Autodesk Fusion 360 part; units mm, degrees
sketch "Sketch1" plane through (0, 0, 0) normal (0, 0, 1) x (1, 0, 0)
  line L0 (0, 0) -> (-48, 0)
  line L1 (-48, 0) -> (-48, 48)
  line L2 (-48, 48) -> (0, 48)
  line L3 (0, 48) -> (0, 0)
  dimension "d1" = 48
  dimension "d2" = 48
extrude "Extrude1" add sketch "Sketch1" along normal blind 10
sketch "Sketch2" plane through (0, 0, 10) normal (0, 0, 1) x (-1, 0, 0)
  line L0 (0, -48) -> (48, -48)
  line L1 (48, -48) -> (48, 0)
  line L2 (48, 0) -> (0, 0)
  line L3 (0, 0) -> (0, -48)
  line L4 (34.25, -13.75) -> (13.75, -13.75)
  line L5 (13.75, -13.75) -> (13.75, -34.25)
  line L6 (13.75, -34.25) -> (34.25, -34.25)
  line L7 (34.25, -34.25) -> (34.25, -13.75)
  line L8 (34.25, -13.75) -> (13.75, -34.25) construction
  line L9 (13.75, -13.75) -> (34.25, -34.25) construction
  point P0 (24, -24)
  dimension "d5" = 20.5
  dimension "d6" = 20.5
extrude "Extrude2" cut sketch "Sketch2" against normal blind 7 contours L4 L5 L6 L7
sketch "Sketch3" plane through (0, 0, 10) normal (0, 0, 1) x (-1, 0, 0)
  line L0 (13.75, -13.75) -> (34.25, -13.75)
  line L1 (34.25, -13.75) -> (34.25, -34.25)
  line L2 (34.25, -34.25) -> (13.75, -34.25)
  line L3 (13.75, -34.25) -> (13.75, -13.75)
  line L4 (0, -48) -> (48, -48)
  line L5 (48, -48) -> (48, 0)
  line L6 (48, 0) -> (0, 0)
  line L7 (0, 0) -> (0, -48)
sketch "Sketch4" plane through (0, 0, 0) normal (1, 0, 0) x (0, 1, 0)
  line L0 (0, 0) -> (48, 0)
  line L1 (48, 0) -> (48, 10)
  line L2 (48, 10) -> (0, 10)
  line L3 (0, 10) -> (0, 0)
  line L4 (0, 10) -> (18, 10)
  line L5 (18, 10) -> (18, 6.5)
  line L6 (18, 6.5) -> (0, 6.5)
  line L7 (0, 6.5) -> (0, 10)
  circle A0 centre (18, 6.5) radius 2
  dimension "d9" = 18
  dimension "d10" = 3.5
  dimension "d11" = 4
extrude "Extrude3" cut sketch "Sketch4" against normal blind 15 contours L5 L6 A0 | L5 L6 A0
fillet "Fillet1" radius 4 1 edges at (0, 48, 5)
fillet "Fillet2" radius 4 1 edges at (0, 0, 5)
fillet "Fillet3" radius 4 2 edges at (-48, 48, 5) (-48, 0, 5)
sketch "Sketch5" plane through (0, 0, 10) normal (0, 0, 1) x (-1, 0, 0)
  line L0 (13.75, -13.75) -> (11.25, -13.75)
  line L1 (11.25, -13.75) -> (11.25, -11.25)
  line L2 (11.25, -11.25) -> (13.75, -11.25)
  line L3 (13.75, -11.25) -> (13.75, -13.75)
  line L4 (11.25, -11.25) -> (36.75, -11.25)
  line L5 (36.75, -11.25) -> (36.75, -36.75)
  line L6 (36.75, -36.75) -> (11.25, -36.75)
  line L7 (11.25, -36.75) -> (11.25, -11.25)
  circle A0 centre (36.75, -36.75) radius 1.6
  circle A1 centre (11.25, -36.75) radius 1.6
  circle A2 centre (11.25, -11.25) radius 1.6
  circle A3 centre (36.75, -11.25) radius 1.6
  point P0 (13.75, -13.75)
  dimension "d20" = 2.5
  dimension "d21" = 2.5
  dimension "d22" = 25.5
  dimension "d23" = 25.5
  dimension "d24" = 3.2
  dimension "d25" = 3.2
  dimension "d26" = 3.2
  dimension "d27" = 3.2
extrude "Extrude4" cut sketch "Sketch5" against normal blind 2 contours L1 L2 L4 L7 A2 | L1 L2 L4 L7 A2 | L6 L7 A1 | L6 L7 A1 | L4 L5 A3 | L4 L5 A3 | L5 L6 A0 | L5 L6 A0
sketch "Sketch6" plane through (0, 0, 0) normal (0, 0, -1) x (1, 0, 0)
  arc A0 (-44, 0) -> (-48, -4) centre (-44, -4) ccw
  line L0 (-48, -4) -> (-48, -44)
  arc A1 (-48, -44) -> (-44, -48) centre (-44, -44) ccw
  line L1 (-44, -48) -> (-4, -48)
  arc A2 (-4, -48) -> (0, -44) centre (-4, -44) ccw
  line L2 (0, -44) -> (0, -4)
  arc A3 (0, -4) -> (-4, 0) centre (-4, -4) ccw
  line L3 (-4, 0) -> (-44, 0)
  line L4 (0, 0) -> (-4, 0)
  line L5 (0, -4) -> (0, 0)
  circle A4 centre (-4, -44) radius 1.5
  circle A5 centre (-44, -44) radius 1.5
  circle A6 centre (-44, -4) radius 1.5
  circle A7 centre (-4, -4) radius 1.5
  dimension "d30" = 4
  dimension "d31" = 40
  dimension "d33" = 3
  dimension "d34" = 3
  dimension "d35" = 3
  dimension "d36" = 3
extrude "Extrude5" add sketch "Sketch6" along normal blind 2 contours A4 | A5 | A6 | A7
sketch "Sketch7" plane through (0, 0, 10) normal (0, 0, 1) x (-1, 0, 0)
  line L0 (0, 0) -> (4, 0)
  line L1 (4, 0) -> (4, -4)
  line L2 (4, -4) -> (0, -4)
  line L3 (0, -4) -> (0, 0)
  line L4 (4, -4) -> (44, -4)
  line L5 (44, -4) -> (44, -44)
  line L6 (44, -44) -> (4, -44)
  line L7 (4, -44) -> (4, -4)
  circle A0 centre (4, -4) radius 1.6
  circle A1 centre (44, -4) radius 1.6
  circle A2 centre (4, -44) radius 1.6
  circle A3 centre (44, -44) radius 1.6
  dimension "d39" = 4
  dimension "d40" = 4
  dimension "d41" = 40
  dimension "d42" = 40
  dimension "d43" = 3.2
  dimension "d44" = 3.2
  dimension "d45" = 3.2
  dimension "d46" = 3.2
extrude "Extrude6" cut sketch "Sketch7" against normal blind 2 contours L1 L4 A0 | L1 L2 A0 | L2 L7 A0 | L4 L7 A0 | L4 L5 A1 | L4 L5 A1 | L6 L7 A2 | L6 L7 A2 | L5 L6 A3 | L5 L6 A3
extrude "Extrude7" cut 4 faces at (-44.3721, 3.7344, -2) (-4.5584, 4.2485, -2) (-4.4413, 44.3401, -2) (-43.9601, 44.4654, -2) along direction (0, 0, 1) blind 2
sketch "Sketch8" plane through (0, 0, 0) normal (0, 0, -1) x (1, 0, 0)
  arc A0 (-44, 0) -> (-48, -4) centre (-44, -4) ccw
  line L0 (-48, -4) -> (-48, -44)
  arc A1 (-48, -44) -> (-44, -48) centre (-44, -44) ccw
  line L1 (-44, -48) -> (-4, -48)
  arc A2 (-4, -48) -> (0, -44) centre (-4, -44) ccw
  line L2 (0, -44) -> (0, -4)
  arc A3 (0, -4) -> (-4, 0) centre (-4, -4) ccw
  line L3 (-4, 0) -> (-44, 0)
  line L4 (0, 0) -> (-4, 0)
  line L5 (-4, 0) -> (-4, -4)
  line L6 (-4, -4) -> (0, -4)
  line L7 (0, -4) -> (0, 0)
  line L8 (-4, -4) -> (-44, -4)
  line L9 (-44, -4) -> (-44, -44)
  line L10 (-44, -44) -> (-4, -44)
  line L11 (-4, -44) -> (-4, -4)
  circle A4 centre (-24, -4) radius 1.5
  circle A5 centre (-24, -44) radius 1.5
  circle A6 centre (-4, -24) radius 1.5
  circle A7 centre (-44, -24) radius 1.5
  dimension "d51" = 4
  dimension "d52" = 40
  dimension "d53" = 40
  dimension "d54" = 3
  dimension "d55" = 3
  dimension "d56" = 3
  dimension "d57" = 3
extrude "Extrude8" add sketch "Sketch8" along normal blind 2 contours L8 A4 | L8 A4 | L11 A6 | L11 A6 | L9 A7 | L9 A7 | L10 A5 | L10 A5
sketch "Sketch9" plane through (0, 0, 10) normal (0, 0, 1) x (-1, 0, 0)
  circle A0 centre (4, -4) radius 1.7
  dimension "d60" = 3.4
extrude "Extrude9" cut sketch "Sketch9" against normal blind 2
sketch "Sketch10" plane through (0, 0, 10) normal (0, 0, 1) x (-1, 0, 0)
  circle A0 centre (4, -44) radius 1.7
  arc A1 (0, -44) -> (4, -48) centre (4, -44) ccw
  dimension "d63" = 3.4
extrude "Extrude10" cut sketch "Sketch10" against normal blind 2
sketch "Sketch11" plane through (0, 0, 10) normal (0, 0, 1) x (-1, 0, 0)
  circle A0 centre (44, -4) radius 1.7
  dimension "d66" = 3.4
extrude "Extrude11" cut sketch "Sketch11" against normal blind 2
sketch "Sketch12" plane through (0, 0, 10) normal (0, 0, 1) x (-1, 0, 0)
  circle A0 centre (44, -44) radius 1.7
  dimension "d69" = 3.4
extrude "Extrude12" cut sketch "Sketch12" against normal blind 2
sketch "Sketch13" plane through (0, 0, 10) normal (0, 0, 1) x (-1, 0, 0)
  circle A0 centre (11.25, -11.25) radius 1.7
  circle A1 centre (11.25, -11.25) radius 1.6
  dimension "d72" = 3.4
extrude "Extrude13" cut sketch "Sketch13" against normal blind 2
sketch "Sketch14" plane through (0, 0, 10) normal (0, 0, 1) x (-1, 0, 0)
  circle A0 centre (36.75, -11.25) radius 1.7
  circle A1 centre (36.75, -11.25) radius 1.6
  dimension "d75" = 3.4
extrude "Extrude14" cut sketch "Sketch14" against normal blind 2
sketch "Sketch15" plane through (0, 0, 10) normal (0, 0, 1) x (-1, 0, 0)
  circle A0 centre (36.75, -36.75) radius 1.7
  circle A1 centre (36.75, -36.75) radius 1.6
  dimension "d78" = 3.4
extrude "Extrude15" cut sketch "Sketch15" against normal blind 2
sketch "Sketch16" plane through (0, 0, 10) normal (0, 0, 1) x (-1, 0, 0)
  circle A0 centre (11.25, -36.75) radius 1.7
  circle A1 centre (11.25, -36.75) radius 1.6
  dimension "d81" = 3.4
extrude "Extrude16" cut sketch "Sketch16" against normal blind 2
Part model, mm, in its own coordinate system. A direction names the side the tool comes from. Round coordinates to 2 decimals unless told otherwise and drop trailing zeros. Loops run counter-clockwise (first coordinate to the right, second up) from the corner with the lowest first, then second, coordinate; pieces in that order, holes last. Notation, with made-up numbers: (69.5, 67) -> (74.5, 67) arc R10 cw to (74.5, 71) -> close; hole circle Ø3 at (-38.75, 42). An arc over 180 degrees is marked (long way). Use CSV: the item, a comma, the result in double quotes. Start each with the question number.
1) Cut at D-D, the plane z = 6.5. Write the cut outline in (x, y), plus the area to 3 significant figures.
2) Drop flat-ended pins along their axis: P1, Ø1.7, axis at x = -4.5, y = 4.5, coming from the +Z side; P2, Ø6, axis at x = -10.5, y = 9, coming from the -Z side. Give the stop position or say it passes through.
3) Cut at C-C, the plane y = 33.5. Write the cut outline in (x, z).
4) Which spindle directions (+Z, -Z, +X, -X, +Y, -Y) get a long thin tool onto all of the face, cutting with end or side? Do faces 4 (the flat face through (-44, 4, 8)), 5 (the flat face through (-24, 0, 5)), 6 (the cylindrical face through (-25.5, 4.07, -0.99)). Say none if no direction does.
5) Pull direction Y, two halves, no side cores. Call faces 1 (the cylindrical face through (-45.11, 25.01, -0.99)), 2 (the cylindrical face through (-1.141, 46.797, 5.07)), 3 (the flat face through (-24, 13.75, 7)): +Y half, -Y half, draft (parallel to the pull), parting line (faces both ways), or undercut.
6) Cut at A-A, the plane y = 18. Write the cut outline in (x, z), plus the area to 4 significant figures.
7) Wall check: L1, parallel to Y at x = -44, z = 8.65; L2, parallel to X at y = 11.25, z = 8.95; L3, parallel to X at y = 44, z = 8.7. Give the ranges that are in metal, low to high. Write a range as [from, to].
8) Cut at B-B, the plane x = -11.25. Write the cut outline in (y, z).
Determined:
1,outline,"(-48, 4) arc R4 ccw to (-44, 0) -> (-4, 0) arc R4 ccw to (0, 4) -> (0, 16) -> (-13.75, 16) -> (-13.75, 13.75) -> (-34.25, 13.75) -> (-34.25, 34.25) -> (-13.75, 34.25) -> (-13.75, 20) -> (0, 20) -> (0, 44) arc R4 ccw to (-4, 48) -> (-44, 48) arc R4 ccw to (-48, 44) -> close"
1,area,"1,820 mm2"
2,P1,"stops at z = 8"
2,P2,"stops at z = 0"
3,outline,"(-48, 0) -> (0, 0) -> (0, 10) -> (-13.75, 10) -> (-13.75, 3) -> (-34.25, 3) -> (-34.25, 10) -> (-48, 10) -> close"
4,face 4,"+Z"
4,face 5,"+Z, -Z, +X, -X, -Y"
4,face 6,"-Z"
5,face 1,"parting line"
5,face 2,"+Y half"
5,face 3,"undercut"
6,outline,"(-48, 0) -> (0, 0) -> (0, 4.5) -> (-13.75, 4.5) -> (-13.75, 3) -> (-34.25, 3) -> (-34.25, 10) -> (-48, 10) -> close; (-13.75, 8.5) -> (0, 8.5) -> (0, 10) -> (-13.75, 10) -> close"
6,area,"281.5 mm2"
7,L1,"y = [0, 2.3], [5.7, 42.3], [45.7, 48]"
7,L2,"x = [-48, -38.45], [-35.05, -12.95], [-9.55, 0]"
7,L3,"x = [-48, -45.7], [-42.3, -5.7], [-2.3, 0]"
8,outline,"(0, 0) -> (48, 0) -> (48, 10) -> (38.45, 10) -> (38.45, 8) -> (35.05, 8) -> (35.05, 10) -> (12.95, 10) -> (12.95, 8) -> (9.55, 8) -> (9.55, 10) -> (0, 10) -> close; hole circle Ø4 at (18, 6.5)"
